```python
from build123d import *

# Parameters (mm, degrees)
ESQUISSE1_W                  = 50
ESQUISSE1_H                  = 49.2
BOSS_EXTRU_1_DEPTH           = 5
ESQUISSE4_W                  = 50
ESQUISSE4_H                  = 5
BOSS_EXTRU_3_DEPTH           = 70
ESQUISSE5_R                  = 10
ESQUISSE5_R_2                = 1.25
ENL_V_MAT_EXTRU_1_DEPTH      = 100.099142277
ESQUISSE6_R                  = 11
ENL_V_MAT_EXTRU_2_DEPTH      = 2
ENL_V_MAT_EXTRU_3_DEPTH      = 103.69196658
ENL_V_MAT_EXTRU_3_DEPTH_BACK = 103.69196658
ESQUISSE7_R                  = 2.5
ESQUISSE8_R                  = 2.5
ENL_V_MAT_EXTRU_4_DEPTH      = 103.69196658
ESQUISSE10_R                 = 25
ESQUISSE10_R_2               = 15
BOSS_EXTRU_4_DEPTH           = 30
ESQUISSE12_W                 = 50
ESQUISSE12_H                 = 70
ENL_V_MAT_EXTRU_6_DEPTH      = 39.2


with BuildPart() as part:
    # Esquisse1 → Boss.-Extru.1 (new body)
    with BuildSketch(Plane.XY):
        with Locations((25, 24.6)):
            Rectangle(ESQUISSE1_W, ESQUISSE1_H)
    extrude(amount=BOSS_EXTRU_1_DEPTH)

    # Esquisse4 → Boss.-Extru.3 (add)
    with BuildSketch(Plane.XY.offset(5)):
        with Locations((25, 46.7)):
            Rectangle(ESQUISSE4_W, ESQUISSE4_H)
        with Locations((25, 2.5)):
            Rectangle(ESQUISSE4_W, ESQUISSE4_H)
    extrude(amount=BOSS_EXTRU_3_DEPTH)

    # Esquisse5 → Enlèv. mat.-Extru.1 (cut, through all)
    with BuildSketch(Plane.XY.offset(5)):
        with Locations((25, 24.6)):
            Circle(ESQUISSE5_R)
        with Locations((9.3, 8.9)):
            Circle(ESQUISSE5_R_2)
        with Locations((40.7, 40.3)):
            Circle(ESQUISSE5_R_2)
        with Locations((40.7, 8.9)):
            Circle(ESQUISSE5_R_2)
        with Locations((9.3, 40.3)):
            Circle(ESQUISSE5_R_2)
    extrude(amount=-ENL_V_MAT_EXTRU_1_DEPTH, mode=Mode.SUBTRACT)

    # Esquisse6 → Enlèv. mat.-Extru.2 (cut)
    with BuildSketch(Plane(origin=(0, 0, 0), x_dir=(-1, 0, 0), z_dir=(0, 0, -1))):
        with Locations((-25, 24.6)):
            Circle(ESQUISSE6_R)
    extrude(amount=-ENL_V_MAT_EXTRU_2_DEPTH, mode=Mode.SUBTRACT)

    # Esquisse7 → Enlèv. mat.-Extru.3 (cut, two sides: drawn at the far end of the back side and taken through both)
    with BuildSketch(Plane.XZ.offset(-ENL_V_MAT_EXTRU_3_DEPTH_BACK)):
        with Locations(Location((25, 34, 0), (0, 0, 270))):
            Circle(ESQUISSE7_R)
    extrude(amount=ENL_V_MAT_EXTRU_3_DEPTH + ENL_V_MAT_EXTRU_3_DEPTH_BACK, mode=Mode.SUBTRACT)

    # Esquisse8 → Enlèv. mat.-Extru.4 (cut, through all)
    with BuildSketch(Plane.XZ):
        with Locations(Location((10.4, 60.5, 0), (0, 0, 270))):
            Circle(ESQUISSE8_R)
    extrude(amount=-ENL_V_MAT_EXTRU_4_DEPTH, mode=Mode.SUBTRACT)

    # Esquisse10 → Boss.-Extru.4 (add, symmetric)
    with BuildSketch(Plane(origin=(50, 5, 5), x_dir=(0.7071067811865476, 0, 0.7071067811865475), z_dir=(-0.7071067811865475, 0, 0.7071067811865476))):
        with Locations(Location((21.226499819, 19.6, 0), (0, 0, 231.628284853))):
            Circle(ESQUISSE10_R)
        with Locations((21.226499819, 19.6)):
            Circle(ESQUISSE10_R_2, mode=Mode.SUBTRACT)
    extrude(amount=BOSS_EXTRU_4_DEPTH, both=True)

    # Esquisse12 → Enlèv. mat.-Extru.6 (cut)
    with BuildSketch(Plane(origin=(0, 5, 0), x_dir=(1, 0, 0), z_dir=(0, 1, 0))):
        with Locations((25, -40)):
            Rectangle(ESQUISSE12_W, ESQUISSE12_H)
    extrude(amount=ENL_V_MAT_EXTRU_6_DEPTH, mode=Mode.SUBTRACT)


solid = part.part
```
Build history of the part. All positions in model axes, mm. A direction names the side the tool comes from. Coordinates: 2 decimals unless noted, no trailing zeros. Order: outer loops, then holes, each group sorted by start corner. A loop starts at its lowest first (then second) coordinate and runs counter-clockwise, first axis right, second up. Notation, with made-up numbers: (22.5, 4.25) -> (81.5, 4.25) arc R34 ccw to (81.5, 41.25) -> close; hole circle Ø11 at (52.25, 49.25). An arc over 180 degrees is marked (long way). Answer in a Markdown table with one row per item. Add a question column.
Q1. Band-saw the part on B-B, the plane y = 19. List the corners of the cut face in (x, z), then the cut area to 3 significant figures.
Q2. Wall check: line 1 along Y through (x, z) = (40.7, 3.15); line 2 along Z through (x, y) = (25, 46.35); line 3 along Y through (x, z) = (25, 1.5). Give the ranges that are in metal, low to high. Write a range as [from, to].
Q3. Mould opens along Z. For faces 1 (the face through (86.88, 28.56, 33.05)), 2 (the face through (11.151, 2.465, 58.115)), 3 (the face through (25, 0, 37)) say: +Z half, -Z half, draft (parallel to the pull), parting line (faces both ways), or undercut.
Q4. Band-saw the part on C-C, the plane y = 43. List the corners of the cut face in (x, z), then the cut area to 3 significant figures.
Q5. Band-saw the part on D-D, the plane z = 49.5. Give the number of separate pieces and of enclosed holes in the cut face, then the cut area to 3 significant figures.
Q6. Band-saw the part on A-A, the plane z = 67. List the corners of the cut face in (x, y).
Q7. Drop flat-ended pins along their axis: pin 1 (2 mm diameter, centred on x = 18, y = 7.5, fed in from -Z); pin 2 (6 mm diameter, centred on x = 10.4, z = 60.5, fed in from +Y); pin 3 (15 mm diameter, centred on x = 37, z = 55, fed in from -Y); pin 4 (4.5 mm diameter, centred on x = 25, z = 34, fed in from +Y). Give the stop position or say it passes through.
Q8. Which spindle directions (+Z, -Z, +X, -X, +Y, -Y) get a long thin tool onto all of the face, cutting with end or side? Do faces 4 (the face through (15, 22, 2)), 5 (the face through (43.721, -0.161, 41.147)), 6 (the face through (19, 34, 5)). Say none if no direction does.
Answers follow:
| question | item | result |
|---|---|---|
| 1 | outline | (0, 0) -> (15.53, 0) -> (15.53, 2) -> (16.72, 2) -> (16.72, 5) -> (0, 5) -> close; (33.28, 2) -> (34.47, 2) -> (34.47, 0) -> (50, 0) -> (50, 0.56) -> (68.99, -18.43) -> (76.38, -11.04) -> (50, 15.34) -> (50, 5) -> (33.28, 5) -> close; (53.64, 51.06) -> (96.06, 8.64) -> (103.45, 16.02) -> (61.02, 58.45) -> close |
| 1 | area | 1,120 mm^2 |
| 2 | line 1 | [0, 7.65], [10.15, 39.05], [41.55, 49.2] |
| 2 | line 2 | [0, 31.5], [36.5, 75] |
| 2 | line 3 | [0, 13.6], [35.6, 49.2] |
| 3 | face 1 | parting line |
| 3 | face 2 | undercut |
| 3 | face 3 | draft |
| 4 | outline | (0, 0) -> (50, 0) -> (50, 5) -> (0, 5) -> close; (50, 11.08) -> (74.26, -13.17) -> (98.19, 10.76) -> (55.76, 53.19) -> (50, 47.43) -> close |
| 4 | area | 1,950 mm^2 |
| 5 | separate pieces | 3 |
| 5 | enclosed holes | 0 |
| 5 | area | 1,030 mm^2 |
| 6 | outline | (0, 0) -> (50, 0) -> (50, 5) -> (0, 5) -> close; (0, 44.2) -> (50, 44.2) -> (50, 49.2) -> (0, 49.2) -> close |
| 7 | pin 1 | z = 0 |
| 7 | pin 2 | y = 49.2 |
| 7 | pin 3 | y = 0 |
| 7 | pin 4 | through |
| 8 | face 4 | -Z |
| 8 | face 5 | +Z, -X, -Y |
| 8 | face 6 | +Z, -X |
